The listing builds one solid part. Answer for the finished solid, in the listing's coordinates (mm). A direction names the side the tool comes from. Coordinates: 2 decimals unless noted, no trailing zeros. Loops run counter-clockwise (first coordinate to the right, second up) from the corner with the lowest first, then second, coordinate; pieces in that order, holes last. Notation, with made-up numbers: (59, 76.25) - (73, 76.25) arc R16 ccw to (73, 81.25) - close; hole circle Ø3 at (87, -13). An arc over 180 degrees is marked (long way). Return JSON: item names as keys, results as strings. Group by question number.
1. Which of the six approach directions +Z, -Z, +X, -X, +Y, -Y give full straight-line access (tool end or side, diameter ignored) to faces 4 (the face through (7, 0, 5.7)), 5 (the face through (8, 0, 6.5))?
2. Each of these flat-tipped pins is pushed along its axis until it touches: P1, Ø0.7, axis at y = -5, z = 2, coming from the -X side; P2, Ø2, axis at x = 8, y = -0.5, coming from the -Z side; P3, Ø3, axis at y = 2, z = 5.5, coming from the -X side. Where does it stop, or does it pass through?
3. Find the intervals of material crossed by line 1 along Z through (x, y) = (6, 3); line 2 along Y through (x, z) = (10.75, 3.25); line 3 along Y through (x, z) = (9, 3.5), in increasing order.
4. Section C-C (y = -2.5) is taken. Write down the section's boundary in (x, z), and give its area (3 significant figures).
5. Section B-B (x = 9.75) is taken. Write down the section's boundary in (y, z).
6. The mould has two halves that part along Y. Classify faces 1 (the face through (12.212, 2.665, 2.81)), 2 (the face through (9.803, 4.743, 3.204)), 3 (the face through (14.624, -2.079, 3.204)): pulls with the +Y half, pulls with the -Y half, needs draft (parallel to the pull), parting line crosses it, or undercut.
Autodesk Inventor part; units mm, degrees
ref_plane "YZ Plane" through (0, 0, 0) normal (1, 0, 0) x (0, 1, 0)
ref_plane "XZ Plane" through (0, 0, 0) normal (0, 1, 0) x (-1, 0, 0)
ref_plane "XY Plane" through (0, 0, 0) normal (0, 0, 1) x (1, 0, 0)
sketch "Boceto1" plane through (0, 0, 0) normal (0, 0, 1) x (1, 0, 0)
  line L0 (8.9411, -4.2344) -> (11.6298, -3.6616)
  line L1 (11.6298, -3.6616) -> (13.3209, -2.1424)
  arc A0 (13.3209, -2.1424) -> (13.9587, -0.9739) centre (11.9843, -0.6546) ccw
  line L2 (13.9587, -0.9739) -> (13.978, -0.8543)
  arc A1 (9.9548, 3.6595) -> (9.2184, 3.8) centre (9.2184, 1.8) ccw
  line L3 (9.9548, 3.6595) -> (11.6833, 2.9749)
  arc A2 (12.6312, 2.1939) -> (11.6833, 2.9749) centre (10.9469, 1.1154) ccw
  line L4 (12.6312, 2.1939) -> (13.688, 0.5435)
  line L5 (14.1, 2.7373) -> (14.1, -1.982) construction
  arc A3 (13.978, -0.8543) -> (13.688, 0.5435) centre (12.0037, -0.535) ccw
  line L6 (-3.2, 5.1465) -> (9.2184, 3.8)
  arc A4 (10.323, 4.5892) -> (9.2779, 4.7994) centre (9.2184, 1.8) ccw
  line L7 (10.323, 4.5892) -> (12.0516, 3.9047)
  arc A5 (13.4734, 2.7331) -> (12.0516, 3.9047) centre (10.9469, 1.1154) ccw
  line L8 (13.4734, 2.7331) -> (14.5302, 1.0827)
  arc A6 (14.9652, -1.0139) -> (14.5302, 1.0827) centre (12.0037, -0.535) ccw
  line L9 (14.9652, -1.0139) -> (14.9459, -1.1335)
  arc A7 (13.9892, -2.8863) -> (14.9459, -1.1335) centre (11.9843, -0.6546) ccw
  line L10 (13.9892, -2.8863) -> (12.0994, -4.584)
  line L11 (12.0994, -4.584) -> (8.8118, -5.2844)
  line L12 (-2.782, 6.107) -> (9.2779, 4.7994)
  line L13 (9.2184, 3.8) -> (-3.2, 5.1465)
  line L14 (-3.2816, 5.1553) -> (-3.2, 5.1465)
  line L15 (8.8118, -4.6408) -> (8.9411, -4.2344)
  line L16 (-3.2816, 5.6583) -> (-2.782, 6.107)
  line L17 (-3.2816, 5.6583) -> (-3.2816, 5.1553)
  line L18 (8.8118, -5.2844) -> (8.8118, -4.6408)
  point P0 (0, 0)
  point P1 (14.1, -0.1)
  point P2 (9.6, 3.8)
  dimension "d1" = 2
  dimension "d2" = 1
extrude "Extrusión1" add sketch "Boceto1" along normal blind 6.5
sketch "Boceto2" plane through (0, 0, 6.5) normal (0, 0, 1) x (1, 0, 0)
  line L0 (7.1, -4.15) -> (7.1, -7.1226) construction
  line L1 (-3.2, 3.2) -> (-3.2, -3.4) construction
  line L2 (-1.4, 3.8) -> (-1.4, 6.2978) construction
  line L3 (14.1, 2.7373) -> (14.1, -1.982) construction
  line L4 (7.1, -4.15) -> (8.5447, -4.3189)
  line L5 (8.5447, -4.3189) -> (11.6298, -3.6616)
  line L6 (11.6298, -3.6616) -> (13.3209, -2.1424)
  line L7 (13.9587, -0.9739) -> (13.978, -0.8543)
  line L8 (9.9548, 3.6595) -> (11.6833, 2.9749)
  line L9 (12.6312, 2.1939) -> (13.688, 0.5435)
  arc A0 (12.6312, 2.1939) -> (11.6833, 2.9749) centre (10.9469, 1.1154) ccw
  arc A1 (9.9548, 3.6595) -> (9.2184, 3.8) centre (9.2184, 1.8) ccw
  arc A2 (13.978, -0.8543) -> (13.688, 0.5435) centre (12.0037, -0.535) ccw
  arc A3 (13.3209, -2.1424) -> (13.9587, -0.9739) centre (11.9843, -0.6546) ccw
  line L10 (-1.6574, 2.7373) -> (-2.4537, 3.981)
  line L11 (-2.4537, 3.981) -> (-3.3251, 4.3261)
  line L12 (-3.3251, 4.3261) -> (-3.2, 5.1465)
  line L13 (-3.2, 5.1465) -> (9.2184, 3.8)
  line L14 (7.1, -4.15) -> (4.0215, -3.7498)
  arc A4 (4.0215, -3.7498) -> (-1.6574, 2.7373) centre (-2.942, -4.1165) ccw
  point P0 (0, 0)
  point P1 (0, 0)
  point P2 (9.6, 3.8)
  point P3 (14.1, -0.1)
  dimension "d7" = 4.15
  dimension "d8" = 10.3
  dimension "d9" = 3.8
  dimension "d10" = 1.8
  dimension "d11" = 11
  dimension "d12" = 7
  dimension "d13" = 2
extrude "Extrusión2" add sketch "Boceto2" against normal blind 0.8
properties part number "Pieza3_Carcasa_3DPrint"
The answers:
{
 "1": {"face 4": "-Z, -X", "face 5": "+Z, +X, -X, +Y, -Y"},
 "2": {"P1": "stops at x = 8.81", "P2": "stops at z = 5.7", "P3": "stops at x = -2.14"},
 "3": {"line 1": "z = 5.7 to 6.5", "line 2": "y = -4.87 to -3.85, 3.34 to 4.42", "line 3": "y = -5.24 to -4.22, 3.82 to 4.83"},
 "4": {"outline": "(3.84, 5.7) - (12.92, 5.7) - (12.92, 0) - (14.35, 0) - (14.35, 6.5) - (3.84, 6.5) - close", "area": "16.5 mm2"},
 "5": {"outline": "(-5.08, 0) - (-4.06, 0) - (-4.06, 5.7) - (3.73, 5.7) - (3.73, 0) - (4.75, 0) - (4.75, 6.5) - (-5.08, 6.5) - close"},
 "6": {"face 1": "undercut", "face 2": "pulls with the +Y half", "face 3": "pulls with the -Y half"}
}
